Input: part model. Units: mm. Frame: model coordinates. Coordinates: 2 decimals unless noted, no trailing zeros. Order: outer loops, then holes, each group sorted by start corner. A loop starts at its lowest first (then second) coordinate and runs counter-clockwise, first axis right, second up. Notation, with made-up numbers: (24, 83.25) -> (48, 83.25) arc R16 cw to (48, 110.25) -> close; hole circle Ø2 at (-24, 71). An arc over 180 degrees is marked (long way). Use one line per item in the form item = value. Start each with the question number.
1) Pin query (flat end, axial travel): pin 1 (1.5 mm diameter, centred on x = -10, z = 4.5, fed in from -Y); pin 2 (3 mm diameter, centred on y = -55.5, z = 5, fed in from -X); pin 3 (12 mm diameter, centred on x = 55, y = -43, fed in from +Z). Return the tip coordinate at first contact, or that it passes through.
2) Ray query, line 1 along X through (y, z) = (-1.5, 8); line 2 along Y through (x, z) = (38, 9.25); line 3 along Y through (x, z) = (-33, 10). Return the intervals inside material, ascending.
3) Draft query along X for faces 1 (the flat face through (-1, 1, 0)), 2 (the cylindrical face through (23.633, 51.543, 6.261)), 3 (the cylindrical face through (-2.168, 40.226, 6.261)). Return one class per face: pulls with the +X half, pulls with the -X half, needs draft (parallel to the pull), parting line crosses it, or undercut.
4) Section query B-B on z = 6. Count the separate pieces of the cut face and the enclosed holes in it, then the cut area to 3 significant figures.
5) Section query A-A on x = 0. Output: boundary loops of the cut face in (y, z).
from build123d import *

# Parameters (mm, degrees)
F0_R     = 75
F0_R_2   = 8.1306454005
F0_R_3   = 10
F0_R_4   = 8.004103626
F0_R_5   = 8.2498069198
F0_R_6   = 7.9610699334
F1_DEPTH = 12.7


# Not quite as in the source:
# - a fillet or chamfer that OpenCascade refuses, or shapes differently, is made with other operations: its cross-section is extruded or revolved along the edge and cut away or added
# - the program builds the solid bodies; features that only make, move or delete a surface that nothing else refers to are left out


with BuildPart() as f1:
    # F0 (on Top) → F1 (new body)
    with BuildSketch(Plane.XY):
        Circle(F0_R)
        with Locations((-26.2292288244, -59.023771435)):
            Circle(F0_R_2, mode=Mode.SUBTRACT)
        with Locations((-50, -0.0119686127)):
            Circle(F0_R_3, mode=Mode.SUBTRACT)
        with Locations((-35.3553390593, -35.367307672)):
            Circle(F0_R_3, mode=Mode.SUBTRACT)
        with Locations((0, -50.0119686127)):
            Circle(F0_R_3, mode=Mode.SUBTRACT)
        with Locations((35.3553390593, -35.367307672)):
            Circle(F0_R_3, mode=Mode.SUBTRACT)
        with Locations((60.637563467, -22.0063943416)):
            Circle(F0_R_4, mode=Mode.SUBTRACT)
        with Locations((50, -0.0119686127)):
            Circle(F0_R_3, mode=Mode.SUBTRACT)
        with Locations((-58.0026507378, 24.9211471528)):
            Circle(F0_R_5, mode=Mode.SUBTRACT)
        with Locations((-35.3553390593, 35.3433704467)):
            Circle(F0_R_3, mode=Mode.SUBTRACT)
        with Locations((35.3553390593, 35.3433704467)):
            Circle(F0_R_3, mode=Mode.SUBTRACT)
        with Locations((0, 49.9880313873)):
            Circle(F0_R_3, mode=Mode.SUBTRACT)
        with Locations((25.3583583981, 59.3152455986)):
            Circle(F0_R_6, mode=Mode.SUBTRACT)
    extrude(amount=F1_DEPTH)

    # F2: fillet of radius 12.7 on 1 edges, made by hand

    # F2_s1 → F2_t2 (revolve, cut)
    with BuildSketch(Plane.XZ):
        with BuildLine():
            ThreePointArc((75, 0), (71.2802561211, 8.9802561211), (62.3, 12.7))
            Line((62.3, 12.7), (75, 12.7))
            Line((75, 12.7), (75, 0))
        make_face()
    revolve(axis=Axis((0, 0, 12.7), (0, 0, 1)), mode=Mode.SUBTRACT)


solid = f1.part
Answers below:
q1.pin_1 = -73.78
q1.pin_2 = -50.78
q1.pin_3 = 12.61
q2.line_1 = -72.15 to -59.89, -40.11 to 40.11, 59.89 to 72.15
q2.line_2 = -59.98 to -45.01, -25.72 to 25.7, 44.99 to 59.98
q2.line_3 = -54.52 to -45.09, -25.65 to 25.62, 45.06 to 61.88
q3.face_1 = needs draft
q3.face_2 = undercut
q3.face_3 = undercut
q4.separate_pieces = 1
q4.enclosed_holes = 12
q4.area = 13,600 mm^2
q5.outline = (-75, 0) -> (-60.01, 0) -> (-60.01, 12.7) -> (-62.3, 12.7) arc R12.7 ccw to start; (-40.01, 0) -> (39.99, 0) -> (39.99, 12.7) -> (-40.01, 12.7) -> close; (59.99, 0) -> (75, 0) arc R12.7 ccw to (62.3, 12.7) -> (59.99, 12.7) -> close
